from build123d import *

# Parameters (mm, degrees)
BOSS_EXTRUDE1_DEPTH = 100
SKETCH2_R           = 1.5
CUT_EXTRUDE1_DEPTH  = 148.692247596
SKETCH3_R           = 2.5
CUT_EXTRUDE2_DEPTH  = 158.165517847
FILLET1_R           = 10


with BuildPart() as part:
    # Sketch1 → Boss-Extrude1 (new body)
    with BuildSketch(Plane.XY):
        with BuildLine():
            Line((-1, 25), (1, 25))
            Line((1, 25), (1, -42))
            ThreePointArc((1, -42), (-0.464466094, -45.535533906), (-4, -47))
            Line((-4, -47), (-99, -47))
            Line((-99, -47), (-99, -45))
            Line((-99, -45), (-6, -45))
            ThreePointArc((-6, -45), (-2.464466094, -43.535533906), (-1, -40))
            Line((-1, -40), (-1, 25))
        make_face()
    extrude(amount=BOSS_EXTRUDE1_DEPTH)

    # Sketch2 → Cut-Extrude1 (cut, through all)
    with BuildSketch(Plane.ZY.offset(1)):
        with Locations(Location((19, 4, 0), (0, 0, 270))):
            Circle(SKETCH2_R)
        with Locations(Location((31, 4, 0), (0, 0, 270))):
            Circle(SKETCH2_R)
        with Locations(Location((31, 17, 0), (0, 0, 270))):
            Circle(SKETCH2_R)
        with Locations(Location((19, 17, 0), (0, 0, 270))):
            Circle(SKETCH2_R)
        with Locations(Location((81, 17, 0), (0, 0, 90))):
            Circle(SKETCH2_R)
        with Locations(Location((69, 17, 0), (0, 0, 90))):
            Circle(SKETCH2_R)
        with Locations(Location((69, 4, 0), (0, 0, 90))):
            Circle(SKETCH2_R)
        with Locations(Location((81, 4, 0), (0, 0, 90))):
            Circle(SKETCH2_R)
    extrude(amount=-CUT_EXTRUDE1_DEPTH, mode=Mode.SUBTRACT)

    # Sketch3 → Cut-Extrude2 (cut, through all)
    with BuildSketch(Plane(origin=(0, -45, 0), x_dir=(1, 0, 0), z_dir=(0, 1, 0))):
        with Locations(Location((-21.704136641, -32.22, 0), (0, 0, 180))):
            Circle(SKETCH3_R)
        with Locations(Location((-21.704136641, -67.78, 0), (0, 0, 180))):
            Circle(SKETCH3_R)
        with Locations(Location((-52.5, -85.56, 0), (0, 0, 180))):
            Circle(SKETCH3_R)
        with Locations(Location((-83.295863359, -67.78, 0), (0, 0, 180))):
            Circle(SKETCH3_R)
        with Locations(Location((-83.295863359, -32.22, 0), (0, 0, 180))):
            Circle(SKETCH3_R)
        with Locations(Location((-52.5, -14.44, 0), (0, 0, 180))):
            Circle(SKETCH3_R)
    extrude(amount=-CUT_EXTRUDE2_DEPTH, mode=Mode.SUBTRACT)

    # Fillet1
    fillet1_edges = [part.edges().sort_by_distance(p)[0] for p in [
        (-99, -46, 0),
        (-99, -46, 100),
        (0, 25, 100),
        (0, 25, 0),
    ]]
    fillet(fillet1_edges, radius=FILLET1_R)


solid = part.part
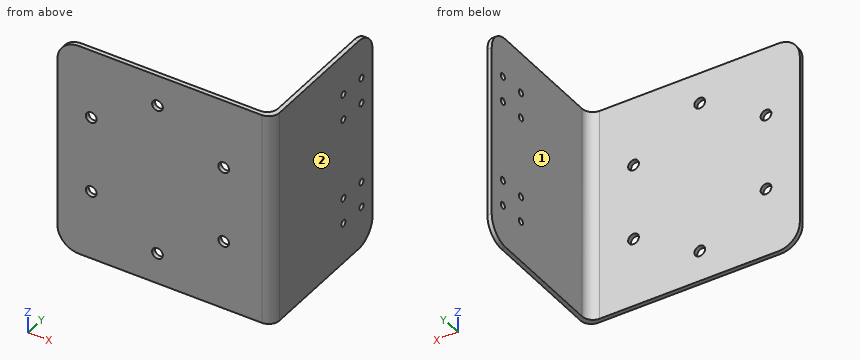
Input: part model. Units: mm. Frame: model coordinates. Face numbers are marked on the shaded views. A direction names the side the tool comes from. Round coordinates to 2 decimals unless told otherwise and drop trailing zeros. Write each loop counter-clockwise with the first axis right and the second up, starting at its lowest first coordinate (ties: lowest second). Pieces come first, ordered by that corner, then holes.
1) Ray query, L1, parallel to Z at x = 0, y = 4; L2, parallel to X at y = -46, z = 32; L3, parallel to Y at x = 0, z = 81. Return the intervals inside material, ascending.
2) Cut plane D-D (y = 17). Return the cut outline in (x, z).
3) Reachability of the marked faces 1 and 2 from +Z, -Z, +X, -X, +Y, -Y: full face, straight path, thin tool, end or side. Return the list, or none.
4) Cut plane B-B (z = 81). Return the cut outline in (x, y).
5) Cut plane C-C (z = 36.5). Return the cut outline in (x, y).
6) Cut plane A-A (y = 4). Return the cut outline in (x, z), then the cut area to 3 significant figures.
7) Contact query for flat-ended pins moving along their axis: P1, Ø1.8, axis at y = 17, z = 81, coming from the +X side; P2, Ø3, axis at y = -19.5, z = 30, coming from the -X side; P3, Ø10, axis at x = -66.5, z = 27, coming from the +Y side. Output: stop coordinate, or through.
Geometry says:
1. L1: z = 0 to 17.5, 20.5 to 29.5, 32.5 to 67.5, 70.5 to 79.5, 82.5 to 100
1. L2: x = -99 to -85.79, -80.81 to -24.19, -19.21 to -1
1. L3: y = -45 to 2.5, 5.5 to 15.5, 18.5 to 25
2. outline: (-1, 0.2) - (1, 0.2) - (1, 17.5) - (-1, 17.5) - close; (-1, 20.5) - (1, 20.5) - (1, 29.5) - (-1, 29.5) - close; (-1, 32.5) - (1, 32.5) - (1, 67.5) - (-1, 67.5) - close; (-1, 70.5) - (1, 70.5) - (1, 79.5) - (-1, 79.5) - close; (-1, 82.5) - (1, 82.5) - (1, 99.8) - (-1, 99.8) - close
3. face 1: +Z, -Z, -X, +Y
3. face 2: +Z, -Z, +X, +Y, -Y
4. outline: (-99, -47) - (-4, -47) arc R5 ccw to (1, -42) - (1, 2.5) - (-1, 2.5) - (-1, -40) arc R5 cw to (-6, -45) - (-99, -45) - close; (-1, 5.5) - (1, 5.5) - (1, 15.5) - (-1, 15.5) - close; (-1, 18.5) - (1, 18.5) - (1, 25) - (-1, 25) - close
5. outline: (-99, -47) - (-4, -47) arc R5 ccw to (1, -42) - (1, 25) - (-1, 25) - (-1, -40) arc R5 cw to (-6, -45) - (-99, -45) - close
6. outline: (-1, 0) - (1, 0) - (1, 17.5) - (-1, 17.5) - close; (-1, 20.5) - (1, 20.5) - (1, 29.5) - (-1, 29.5) - close; (-1, 32.5) - (1, 32.5) - (1, 67.5) - (-1, 67.5) - close; (-1, 70.5) - (1, 70.5) - (1, 79.5) - (-1, 79.5) - close; (-1, 82.5) - (1, 82.5) - (1, 100) - (-1, 100) - close
6. area: 176 mm2
7. P1: passes through
7. P2: stops at x = -1
7. P3: stops at y = -45
